```python
from build123d import *

# Parameters (mm, degrees)
F1_DEPTH = 44
F5_DEPTH = 25
F6_DEPTH = 25


with BuildPart() as f1:
    # F0 (on Front) → F1 (new body, symmetric)
    with BuildSketch(Plane.XZ):
        Polygon((-68, 0), (-33, 0), (-33, 3), (-33, 16), (-68, 16), align=None)
        Polygon((-33, 16), (-33, 3), (33, 3), (33, 16), (33, 17), (-33, 17), align=None)
        Polygon((33, 16), (33, 3), (33, 0), (68, 0), (68, 16), align=None)
    extrude(amount=F1_DEPTH, both=True)

    # F3 (on offset) → F5 (cut)
    with BuildSketch(Plane.XY.offset(16)):
        with BuildLine():
            ThreePointArc((55, 25), (46.4644660941, 28.5355339059), (50, 20))
            ThreePointArc((50, 20), (53.5355339059, 21.4644660941), (55, 25))
        make_face()
        with BuildLine():
            ThreePointArc((55, -25), (53.5355339059, -21.4644660941), (50, -20))
            ThreePointArc((50, -20), (46.4644660941, -28.5355339059), (55, -25))
        make_face()
    extrude(amount=-F5_DEPTH, mode=Mode.SUBTRACT)

    # F4 (on face) → F6 (cut)
    with BuildSketch(Plane.XY.offset(16)):
        with BuildLine():
            ThreePointArc((-45, -27.5), (-46.4644660941, -23.9644660941), (-50, -22.5))
            ThreePointArc((-50, -22.5), (-53.5355339059, -31.0355339059), (-45, -27.5))
        make_face()
        with BuildLine():
            ThreePointArc((-45, 27.5), (-53.5355339059, 31.0355339059), (-50, 22.5))
            ThreePointArc((-50, 22.5), (-46.4644660941, 23.9644660941), (-45, 27.5))
        make_face()
    extrude(amount=-F6_DEPTH, mode=Mode.SUBTRACT)


solid = f1.part
```
Read the model definition and answer for the solid it produces. Units are mm, in the model's axes. A direction names the side the tool comes from. Round coordinates to 2 decimals unless told otherwise and drop trailing zeros. Loops run counter-clockwise (first coordinate to the right, second up) from the corner with the lowest first, then second, coordinate; pieces in that order, holes last. Notation, with made-up numbers: (30.25, -7) -> (52.25, -7) arc R20 ccw to (52.25, 31) -> close; hole circle Ø11 at (23.5, -30.75). An arc over 180 degrees is marked (long way). One line per item, written item: value.
1) Consider L1, parallel to Y at x = 50, z = 8.5; L2, parallel to Y at x = -50, z = 4.25; L3, parallel to X at y = 27.5, z = 7.5. Determine where each line is inside the solid, lowest interval first. Write a range as [from, to].
Answer list:
L1: y = [-44, -30], [-20, 20], [30, 44]
L2: y = [-44, -32.5], [-22.5, 22.5], [32.5, 44]
L3: x = [-68, -55], [-45, 45.67], [54.33, 68]
2) A cutting plane is placed at A-A (x = 48.5). Determine the outline of the cut face in (y, z).
Answer list:
outline: (-44, 0) -> (-29.77, 0) -> (-29.77, 16) -> (-44, 16) -> close; (-20.23, 0) -> (20.23, 0) -> (20.23, 16) -> (-20.23, 16) -> close; (29.77, 0) -> (44, 0) -> (44, 16) -> (29.77, 16) -> close
3) A cutting plane is placed at B-B (z = 7.5). Determine the outline of the cut face in (x, y), and give its area (3 significant figures).
Answer list:
outline: (-68, -44) -> (68, -44) -> (68, 44) -> (-68, 44) -> close; hole circle Ø10 at (-50, -27.5); hole circle Ø10 at (-50, 27.5); hole circle Ø10 at (50, -25); hole circle Ø10 at (50, 25)
area: 11,700 mm²
4) The mould has two halves that part along X. Classify faces 6 (the face through (-1, -44, 9)), 7 (the face through (-33, -1, 1)), 8 (the face through (-68, -1, 8)): pulls with the +X half, pulls with the -X half, needs draft (parallel to the pull), parting line crosses it, or undercut.
Answer list:
face 6: needs draft
face 7: undercut
face 8: pulls with the -X half
5) A cutting plane is placed at C-C (y = -6.5). Determine the outline of the cut face in (x, z).
Answer list:
outline: (-68, 0) -> (-33, 0) -> (-33, 3) -> (33, 3) -> (33, 0) -> (68, 0) -> (68, 16) -> (33, 16) -> (33, 17) -> (-33, 17) -> (-33, 16) -> (-68, 16) -> close
6) A cutting plane is placed at D-D (x = 13). Determine the outline of the cut face in (y, z), and give its area (3 significant figures).
Answer list:
outline: (-44, 3) -> (44, 3) -> (44, 17) -> (-44, 17) -> close
area: 1,230 mm²
7) For faces 1 (the face through (-50, -1, 16)), 2 (the face through (51, -1, 16)), 3 (the face through (33, -1, 2)), 4 (the face through (-1, 44, 9)), 5 (the face through (50, -1, 0)), determine the directions among +Z, -Z, +X, -X, +Y, -Y from which every point of the face is accessible in a straight line to the end or side of a thin tool.
Answer list:
face 1: +Z, -X, +Y, -Y
face 2: +Z, +X, +Y, -Y
face 3: -Z, +Y, -Y
face 4: +Z, -Z, +X, -X, +Y
face 5: -Z, +X, -X, +Y, -Y
8) Flat-ended cylindrical pins translate along their axes: P1, Ø1, axis at x = 0.5, y = 19.5, coming from the -Z side; P2, Ø8, axis at x = 50, y = -25, coming from the +Z side; P3, Ø17.5, axis at x = 52, y = 11.5, coming from the +Z side; P4, Ø0.8, axis at y = -15.5, z = 16.5, coming from the +X side. Find the tip coordinate at first contact, or state that the pin passes through.
Answer list:
P1: stops at z = 3
P2: passes through
P3: stops at z = 16
P4: stops at x = 33
